For this review, take the finished solid that the model builds, in its own axes (mm). A direction names the side the tool comes from. Coordinates: 2 decimals unless noted, no trailing zeros. Loops run counter-clockwise (first coordinate to the right, second up) from the corner with the lowest first, then second, coordinate; pieces in that order, holes last. Notation, with made-up numbers: M 46,38 L 89,38 A18 ccw 89,64 Z; hole C 73.5,-23 d2. An arc over 180 degrees is marked long. Use one line per item in the form item = value.
```python
from build123d import *

# Parameters (mm, degrees)
F0_R     = 10.95
F1_DEPTH = 6.6


with BuildPart() as f1:
    # F0 (on Top) → F1 (new body)
    with BuildSketch(Plane.XY):
        with BuildLine():
            Line((-22.483416, -6.533214), (-23.511816, -25.926714))
            ThreePointArc((-23.511816, -25.926714), (-20.762047, -28.176895), (-17.79831, -30.136691))
            Line((-17.79831, -30.136691), (-0.734302, -23.401873))
            Line((-0.734302, -23.401873), (17.39222, -30.372861))
            ThreePointArc((17.39222, -30.372861), (20.381994, -28.45302), (23.161716, -26.239949))
            Line((23.161716, -26.239949), (22.029592, -7.929939))
            Line((22.029592, -7.929939), (34.260799, 7.155253))
            ThreePointArc((34.260799, 7.155253), (33.358812, 10.591961), (32.113038, 13.919511))
            Line((32.113038, 13.919511), (14.349339, 18.500901))
            Line((14.349339, 18.500901), (3.782119, 34.795051))
            ThreePointArc((3.782119, 34.795051), (0.234886, 34.999212), (-3.314767, 34.84268))
            Line((-3.314767, 34.84268), (-13.161213, 19.364125))
            Line((-13.161213, 19.364125), (-31.923321, 14.349271))
            ThreePointArc((-31.923321, 14.349271), (-33.213645, 11.038741), (-34.161677, 7.614449))
            Line((-34.161677, 7.614449), (-22.483416, -6.533214))
        make_face()
        Polygon((-5.476719, -14.85534), (-6.826935, -22.707532), (-14.30224, -25.464306), (-20.42733, -20.368889), (-19.077114, -12.516697), (-11.601808, -9.759923), align=None, mode=Mode.SUBTRACT)
        Circle(F0_R, mode=Mode.SUBTRACT)
        Polygon((12.435869, -9.799222), (19.486507, -13.509814), (19.798359, -21.471142), (13.059573, -25.721878), (6.008934, -22.011286), (5.697082, -14.049958), align=None, mode=Mode.SUBTRACT)
        Polygon((-23.705785, -0.524213), (-25.609628, 1.891393), (-28.63763, 5.733335), (-25.684357, 13.133212), (-17.799239, 14.275541), (-12.867394, 8.017994), (-15.820667, 0.618117), (-22.303521, -0.321064), align=None, mode=Mode.SUBTRACT)
        Polygon((13.162508, 8.799088), (18.870258, 14.358008), (26.538299, 12.194411), (28.49859, 4.471894), (22.79084, -1.087025), (15.122799, 1.076571), align=None, mode=Mode.SUBTRACT)
        Polygon((-4.300991, 15.237357), (-7.824046, 22.383551), (-3.396788, 29.007702), (4.553524, 28.485661), (8.076579, 21.339467), (3.649322, 14.715315), align=None, mode=Mode.SUBTRACT)
    extrude(amount=F1_DEPTH)


solid = f1.part
```
1. Wall thickness on line 1 along X through (y, z) = (-21, 1); line 2 along Y through (x, z) = (-1, 3.5); line 3 along Y through (x, z) = (0, 3.75): over which ranges is each line inside the solid? List them lowest first. Write a range as from..to.
Computed values:
line_1 = -23.25..-19.67, -6.53..5.97, 19.78..22.84
line_2 = -23.51..-10.9, 10.9..15.02, 28.85..34.99
line_3 = -23.68..-10.95, 10.95..14.95, 28.78..35
2. Tool access review of faces 4 (the face through (8.202, -26.839, 3.254)), 5 (the face through (15.912, -11.629, 3.254)), 6 (the face through (22.604, -17.213, 3.254)): name each direction out of +Z, -Z, +X, -X, +Y, -Y from which nothing blocks a thin tool from reaching the whole face with its end or side.
Computed values:
face_4 = +Z, -Z, -Y
face_5 = +Z, -Z
face_6 = +Z, -Z, +X
3. Consider section C-C on z = 3.5. State how many separate pieces and enclosed holes the cut face has, plus the area to 3 significant figures.
Computed values:
separate_pieces = 1
enclosed_holes = 6
area = 1,480 mm2
4. Consider section A-A on y = -3.5. Write out the cut boundary in (x, z).
Computed values:
outline = M -24.99,0 L -10.38,0 L -10.38,6.6 L -24.99,6.6 Z; M 10.38,0 L 25.62,0 L 25.62,6.6 L 10.38,6.6 Z
5. For pin 1 Ø3 at (x, y) = (25, -23.5) entering from -Z; pin 2 Ø1 at (x, z) = (-6.5, 1) entering from +Y, all flat-tipped, find the tip position at first contact; note any pin that passes through.
Computed values:
pin_1 = through
pin_2 = 30.62
6. Consider section D-D on x = 30. Write out the cut boundary in (y, z), plus the area to 3 significant figures.
Computed values:
outline = M 1.9,0 L 14.46,0 L 14.46,6.6 L 1.9,6.6 Z
area = 82.9 mm2
7. Draft analysis for pull direction X (two halves, no side actions). For faces 1 (the face through (25.685, 1.731, 3.254)), 2 (the face through (23.356, 16.178, 3.254)), 3 (the face through (-28.404, 0.64, 3.254)), state which applies: +X half, -X half, draft (parallel to the pull), parting line (faces both ways), or undercut.
Computed values:
face_1 = undercut
face_2 = +X half
face_3 = -X half
8. Consider section B-B on y = -19. Write out the cut boundary in (x, z), plus the area to 3 significant figures.
Computed values:
outline = M -23.14,0 L -20.19,0 L -20.19,6.6 L -23.14,6.6 Z; M -6.19,0 L 5.89,0 L 5.89,6.6 L -6.19,6.6 Z; M 19.7,0 L 22.71,0 L 22.71,6.6 L 19.7,6.6 Z
area = 119 mm2
